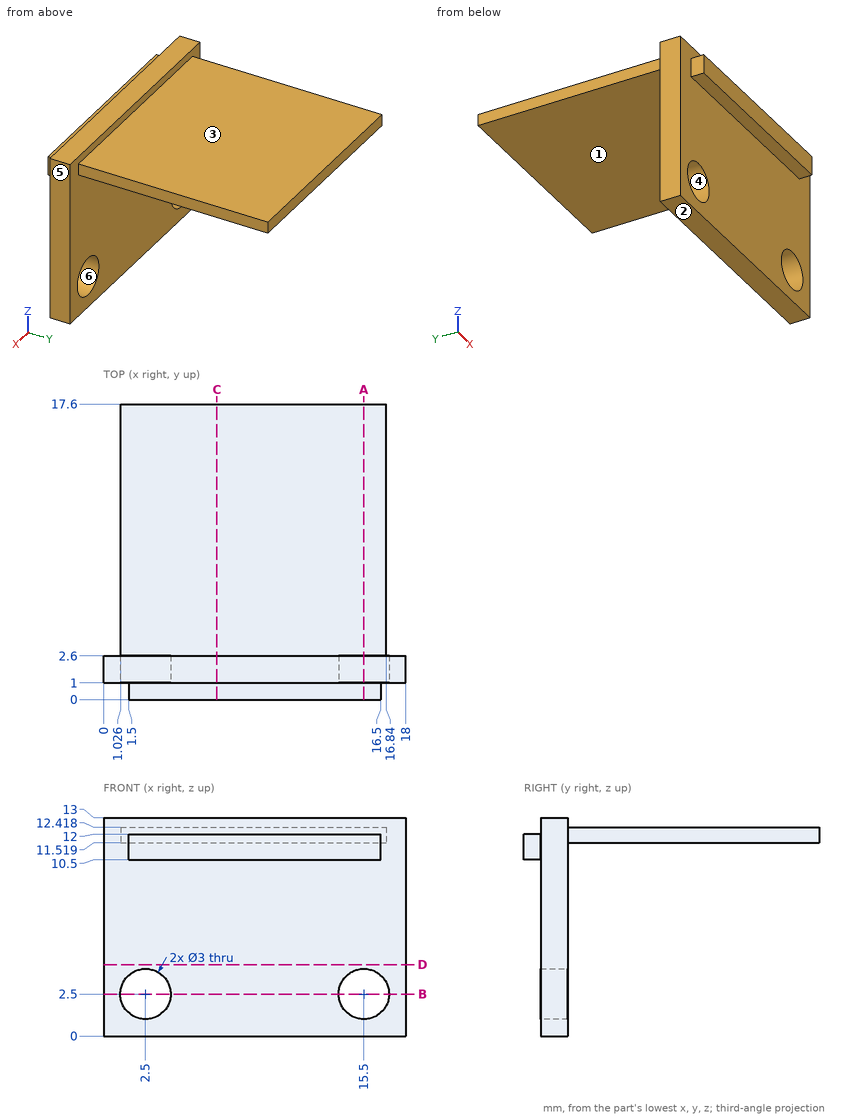
Design review of the part shown in the three views and the two pictorial views. Dimensions are in mm from the part's minimum x, y and z. A direction names the side the tool comes from. Round coordinates to 2 decimals unless told otherwise and drop trailing zeros. Write each loop counter-clockwise with the first axis right and the second up, starting at its lowest first coordinate (ties: lowest second). Pieces come first, ordered by that corner, then holes. Notation, with made-up numbers: (70, -19.5) - (77, -19.5) arc R17 ccw to (77, 11.5) - close; hole circle Ø6 at (16.25, -35). An arc over 180 degrees is marked (long way). Return JSON: item names as keys, results as strings. Group by question number.
Item 1: We need section D-D on z = 4.25. Write out the cut boundary in (x, y).
Item 2: The part is to be moulded in two halves that separate along X. For the marked faces 3, 4, 5 and 6, say which applies: pulls with the +X half, pulls with the -X half, needs draft (parallel to the pull), parting line crosses it, or undercut.
Item 3: We need section B-B on z = 2.5. Write out the cut boundary in (x, y), and give its area (3 significant figures).
Item 4: Machinability: for the marked faces 1 and 2, which of the approach directions +Z, -Z, +X, -X, +Y, -Y give a long, thin tool a straight path to every point of the face, cutting with its end or side? Answer none if there is none.
Item 5: For probe 1 along X at (y, z) = (1.45, 2.5); probe 2 along X at (y, z) = (2.25, 3.5); probe 3 along Z at (x, y) = (16.5, 8), list the stretches that pass through material, from the lowest coordinate up. Write a range as [from, to].
Item 6: We need section A-A on x = 15.5. Write out the cut boundary in (y, z).
Item 7: Insertion check: P1, Ø4, axis at x = 12, y = 10.5, coming from the +Z side; P2, Ø4, axis at x = 16, z = 3, coming from the +Y side; P3, Ø1.1, axis at y = 0.5, z = 11, coming from the +X side; P4, Ø5, axis at y = 9, z = 11.5, coming from the -X side. Each pin has a flat end and moves straight along its axis. Give the tip position at first contact, or say it passes through.
Item 8: We need section C-C on x = 6.75. Write out the cut boundary in (y, z).
Model answer:
{
 "1": {"outline": "(0, 1) - (18, 1) - (18, 2.6) - (0, 2.6) - close"},
 "2": {"face 3": "needs draft", "face 4": "undercut", "face 5": "pulls with the +X half", "face 6": "undercut"},
 "3": {"outline": "(0, 1) - (1, 1) - (1, 2.6) - (0, 2.6) - close; (4, 1) - (14, 1) - (14, 2.6) - (4, 2.6) - close; (17, 1) - (18, 1) - (18, 2.6) - (17, 2.6) - close", "area": "19.2 mm²"},
 "4": {"face 1": "-Z, +X, -X, +Y", "face 2": "-Z, +X, -X, +Y, -Y"},
 "5": {"probe 1": "x = [0, 1], [4, 14], [17, 18]", "probe 2": "x = [0, 1.38], [3.62, 14.38], [16.62, 18]", "probe 3": "z = [11.52, 12.42]"},
 "6": {"outline": "(0, 10.5) - (1, 10.5) - (1, 4) - (2.6, 4) - (2.6, 11.52) - (17.6, 11.52) - (17.6, 12.42) - (2.6, 12.42) - (2.6, 13) - (1, 13) - (1, 12) - (0, 12) - close; (1, 0) - (2.6, 0) - (2.6, 1) - (1, 1) - close"},
 "7": {"P1": "stops at z = 12.42", "P2": "stops at y = 2.6", "P3": "stops at x = 18", "P4": "stops at x = 1.03"},
 "8": {"outline": "(0, 10.5) - (1, 10.5) - (1, 0) - (2.6, 0) - (2.6, 11.52) - (17.6, 11.52) - (17.6, 12.42) - (2.6, 12.42) - (2.6, 13) - (1, 13) - (1, 12) - (0, 12) - close"}
}
